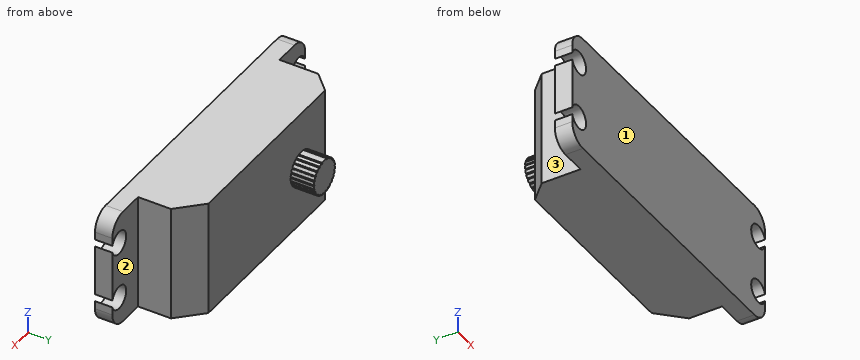
```python
from build123d import *

# Parameters (mm, degrees)
SKETCH_1_W               = 40
SKETCH_1_H               = 12.7
EXTRUDE_1_DEPTH          = 20
EXTRUDE_4_DEPTH          = 3
SKETCH_4_R               = 2
CUT_EXTRUDE_1_DEPTH      = 3
CHAMFER_2_SIZE           = 4
CHAMFER_3_SIZE           = 3
SKETCH_5_R               = 3
EXTRUDE_5_DEPTH          = 4
SKETCH_6_W               = 0.2
SKETCH_6_H               = 4
CUT_EXTRUDE_2_DEPTH      = 0.2
PATTERN_CIRCULAR_1_COUNT = 25


with BuildPart() as part:
    # 草图1 → 凸台-拉伸1 (new body)
    with BuildSketch(Plane.XY):
        Rectangle(SKETCH_1_W, SKETCH_1_H)
    extrude(amount=EXTRUDE_1_DEPTH)

    # 草图3 → 凸台-拉伸4 (add)
    with BuildSketch(Plane.XZ.offset(6.35)):
        with BuildLine():
            Line((-20, 20), (-24.25, 20))
            ThreePointArc((-24.25, 20), (-26.371320344, 19.121320344), (-27.25, 17))
            Line((-27.25, 17), (-27.25, 3))
            ThreePointArc((-27.25, 3), (-26.371320344, 0.878679656), (-24.25, 0))
            Line((-24.25, 0), (-20, 0))
            Line((-20, 0), (-20, 20))
        make_face()
        with BuildLine():
            Line((20, 20), (24.25, 20))
            ThreePointArc((24.25, 20), (26.371320344, 19.121320344), (27.25, 17))
            Line((27.25, 17), (27.25, 3))
            ThreePointArc((27.25, 3), (26.371320344, 0.878679656), (24.25, 0))
            Line((24.25, 0), (20, 0))
            Line((20, 0), (20, 20))
        make_face()
    extrude(amount=-EXTRUDE_4_DEPTH)

    # 草图4 → 切除-拉伸1 (cut)
    with BuildSketch(Plane.XZ.offset(6.35)):
        with Locations((-25.35, 15)):
            Circle(SKETCH_4_R)
        with Locations((-25.35, 5)):
            Circle(SKETCH_4_R)
        with Locations((25.35, 15)):
            Circle(SKETCH_4_R)
        with Locations((25.35, 5)):
            Circle(SKETCH_4_R)
    extrude(amount=-CUT_EXTRUDE_1_DEPTH, mode=Mode.SUBTRACT)

    # 倒角2
    chamfer_2_edges = [part.edges().sort_by_distance(p)[0] for p in [
        (20, 6.35, 10),
    ]]
    chamfer(chamfer_2_edges, length=CHAMFER_2_SIZE)

    # 倒角3
    chamfer_3_edges = [part.edges().sort_by_distance(p)[0] for p in [
        (-20, 6.35, 10),
    ]]
    chamfer(chamfer_3_edges, length=CHAMFER_3_SIZE)

    # 草图5 → 凸台-拉伸5 (add)
    with BuildSketch(Plane(origin=(0, 6.35, 0), x_dir=(1, 0, 0), z_dir=(0, 1, 0))):
        with Locations(Location((-10.25, -10, 0), (0, 0, 90))):
            Circle(SKETCH_5_R)
    extrude_5 = extrude(amount=EXTRUDE_5_DEPTH)

    # 草图6 → 切除-拉伸2 (cut)
    with BuildSketch(Plane.XY.offset(13)):
        with Locations((-10.25, 8.35)):
            Rectangle(SKETCH_6_W, SKETCH_6_H)
    cut_extrude_2 = extrude(amount=-CUT_EXTRUDE_2_DEPTH, mode=Mode.SUBTRACT)

    # 阵列(圆周)1: 凸台-拉伸5, 切除-拉伸2 ×25 about axis
    pattern_circular_1_axis = Axis((-10.25, 10.35, 10), (0, -1, 0))
    add([extrude_5.rotate(pattern_circular_1_axis, i * 360 / PATTERN_CIRCULAR_1_COUNT) for i in range(1, PATTERN_CIRCULAR_1_COUNT)])
    add([cut_extrude_2.rotate(pattern_circular_1_axis, i * 360 / PATTERN_CIRCULAR_1_COUNT) for i in range(1, PATTERN_CIRCULAR_1_COUNT)], mode=Mode.SUBTRACT)


solid = part.part
```
Model file for the job. Use its own axes, mm. Face numbers are marked on the shaded views. A direction names the side the tool comes from. Coordinates: 2 decimals unless noted, no trailing zeros. Loops run counter-clockwise (first coordinate to the right, second up) from the corner with the lowest first, then second, coordinate; pieces in that order, holes last. Notation, with made-up numbers: (73.25, 21) - (132.25, 21) arc R29 cw to (132.25, 41) - close; hole circle Ø5 at (-36.5, -28.75). An arc over 180 degrees is marked (long way). Answer as a JSON object with one key per item and string values. Group by question number.
(1) Tool access for the marked faces 1, 2 and 3: list every direction of +Z, -Z, +X, -X, +Y, -Y with a clear straight run to the whole face (end or side of a thin tool).
(2) Flat gauge pins, fed straight in: pin 1 (6 mm diameter, centred on x = -24, z = 12.5, fed in from +Y); pin 2 (1 mm diameter, centred on y = 2, z = 3.5, fed in from +X); pin 3 (2.5 mm diameter, centred on x = 25.35, z = 15, fed in from +Y); pin 4 (4 mm diameter, centred on y = 6, z = 17, fed in from -X). Where does each tip first touch, or does it go through?
(3) Cut at D-D (x = 2). Give the cut face in (y, z).
(4) Probe line 1 along Z through (x, y) = (25.35, -5.05); line 2 along X through (y, z) = (-4.8, 5); line 3 along Y through (x, z) = (-11, 19). List the from-to ranges inside material, lowest first.
(5) Cut at C-C (x = 25.35). Give the cut face in (y, z), then the cut area to 3 significant figures.
(6) Cut at A-A (z = 3.5). Give the cut face in (x, y), then the cut area to 3 significant figures.
(7) Cut at B-B (y = -4). Give the cut face in (x, z).
Geometry says:
{
 "1": {"face 1": "+Z, -Z, +X, -X, -Y", "face 2": "+Z, -Z, +X, +Y", "face 3": "+Z, -Z, -X, +Y"},
 "2": {"pin 1": "stops at y = -3.35", "pin 2": "stops at x = 20", "pin 3": "passes through", "pin 4": "stops at x = -19.35"},
 "3": {"outline": "(-6.35, 0) - (6.35, 0) - (6.35, 20) - (-6.35, 20) - close"},
 "4": {"line 1": "z = 0.21 to 3, 7 to 13, 17 to 19.79", "line 2": "x = -23.35 to 23.35", "line 3": "y = -6.35 to 6.35"},
 "5": {"outline": "(-6.35, 0.21) - (-3.35, 0.21) - (-3.35, 3) - (-6.35, 3) - close; (-6.35, 7) - (-3.35, 7) - (-3.35, 13) - (-6.35, 13) - close; (-6.35, 17) - (-3.35, 17) - (-3.35, 19.79) - (-6.35, 19.79) - close", "area": "34.7 mm^2"},
 "6": {"outline": "(-27.25, -6.35) - (-26.67, -6.35) - (-26.67, -3.35) - (-27.25, -3.35) - close; (-24.03, -6.35) - (24.03, -6.35) - (24.03, -3.35) - (20, -3.35) - (20, 2.35) - (16, 6.35) - (-17, 6.35) - (-20, 3.35) - (-20, -3.35) - (-24.03, -3.35) - close; (26.67, -6.35) - (27.25, -6.35) - (27.25, -3.35) - (26.67, -3.35) - close", "area": "523 mm^2"},
 "7": {"outline": "(-27.25, 3) arc R3 ccw to (-24.25, 0) - (24.25, 0) arc R3 ccw to (27.25, 3) - (27.25, 4.38) arc R2 cw (long way) to (27.25, 5.62) - (27.25, 14.38) arc R2 cw (long way) to (27.25, 15.62) - (27.25, 17) arc R3 ccw to (24.25, 20) - (-24.25, 20) arc R3 ccw to (-27.25, 17) - (-27.25, 15.62) arc R2 cw (long way) to (-27.25, 14.38) - (-27.25, 5.62) arc R2 cw (long way) to (-27.25, 4.38) - close"}
}
